Check sheet for the modelled part. Datum: model origin and axes. Units: mm. A direction names the side the tool comes from. Round coordinates to 2 decimals unless told otherwise and drop trailing zeros. Write each loop counter-clockwise with the first axis right and the second up, starting at its lowest first coordinate (ties: lowest second). Pieces come first, ordered by that corner, then holes. Notation, with made-up numbers: M 15.5,-14.75 L 67.5,-14.75 A24 ccw 67.5,-3.75 Z; hole C 83.25,76.5 d11. An arc over 180 degrees is marked long. Answer in a Markdown table with one row per item.
```python
from build123d import *

# Parameters (mm, degrees)
SKETCH1_W                    = 127
SKETCH1_H                    = 80.01
BASE_DEPTH                   = 3.81
SKETCH2_W                    = 127
SKETCH2_H                    = 3.81
FRONT_PANELING_DEPTH         = 76.2
SKETCH4_R                    = 1.651
ARDUINO_MOUNTING_HOLES_DEPTH = 107.95368168
STABILITY_STRUT_DEPTH        = 3.81
SKETCH5_R                    = 6.0325
ON_OFF_SWITCH_RECESS_DEPTH   = 130.751494018
SKETCH7_R                    = 3.683
SKETCH7_W                    = 1.778
SKETCH7_H                    = 3.81
POTENTIOMETER_RECESS_DEPTH   = 3.81


with BuildPart() as part:
    # Sketch1 → Base (new body)
    with BuildSketch(Plane(origin=(0, 0, 0), x_dir=(1, 0, 0), z_dir=(0, 1, 0))):
        Rectangle(SKETCH1_W, SKETCH1_H)
    extrude(amount=BASE_DEPTH)

    # Sketch2 → Front Paneling (add)
    with BuildSketch(Plane(origin=(0, 3.81, 0), x_dir=(1, 0, 0), z_dir=(0, 1, 0))):
        with Locations((0, -38.1)):
            Rectangle(SKETCH2_W, SKETCH2_H)
    extrude(amount=FRONT_PANELING_DEPTH)

    # Sketch4 → Arduino Mounting Holes (cut, through all)
    with BuildSketch(Plane(origin=(0, 3.81, 0), x_dir=(1, 0, 0), z_dir=(0, 1, 0))):
        with Locations(Location((-44.45, -28.575, 0), (0, 0, 270))):
            Circle(SKETCH4_R)
        with Locations(Location((-43.18, 19.685, 0), (0, 0, 270))):
            Circle(SKETCH4_R)
        with Locations(Location((31.75, 19.685, 0), (0, 0, 270))):
            Circle(SKETCH4_R)
        with Locations(Location((38.1, -28.575, 0), (0, 0, 270))):
            Circle(SKETCH4_R)
    extrude(amount=-ARDUINO_MOUNTING_HOLES_DEPTH, mode=Mode.SUBTRACT)

    # Sketch3 → Stability Strut (add)
    with BuildSketch(Plane.ZY.offset(55.88)):
        Polygon((36.195, 76.2), (-36.195, 3.81), (-31.115, 3.81), (36.195, 71.12), align=None)
    stability_strut = extrude(amount=STABILITY_STRUT_DEPTH)

    # Mirror Strut: Stability Strut across plane
    add(stability_strut.mirror(Plane(origin=(0, 0, 0), x_dir=(0, 0, 1), z_dir=(1, 0, 0))))

    # Sketch5 → On Off Switch Recess (cut, through all)
    with BuildSketch(Plane.XY.offset(40.005)):
        with Locations((44.45, 40.005)):
            Circle(SKETCH5_R)
    extrude(amount=-ON_OFF_SWITCH_RECESS_DEPTH, mode=Mode.SUBTRACT)

    # Sketch7 → Potentiometer Recess (cut)
    with BuildSketch(Plane.XY.offset(40.005)):
        with Locations((12.7, 40.005)):
            Circle(SKETCH7_R)
        with Locations((20.955, 40.005)):
            Rectangle(SKETCH7_W, SKETCH7_H)
    extrude(amount=-POTENTIOMETER_RECESS_DEPTH, mode=Mode.SUBTRACT)


solid = part.part
```
1. Draft check along Z on faces 1 (the face through (55.88, 37, 0)), 2 (the face through (-1, 39, 40.005)), 3 (the face through (36.488, 1.932, 28.217)), 4 (the face through (57.758, 40.512, 0.507)). Enter one of: +Z half, -Z half, draft (parallel to the pull), parting line (faces both ways), or undercut.
Found:
| item | result |
|---|---|
| face 1 | draft |
| face 2 | +Z half |
| face 3 | undercut |
| face 4 | -Z half |
2. Access from +Z, -Z, +X, -X, +Y, -Y to the whole of each face (thin tool, end or side, straight path). Record for faces 5 (the face through (57.758, 36.994, 2.069)), 6 (the face through (59.69, 37, 0)), 7 (the face through (20.066, 40, 38)), 8 (the face through (-55.88, 37, 0)).
Found:
| item | result |
|---|---|
| face 5 | +X, -X |
| face 6 | -Z, +X, +Y |
| face 7 | +Z, -Z |
| face 8 | -Z, +Y |
3. Section check D-D, the plane x = 44.45. Record the cut outline in (y, z) (1 decimal).
Found:
| item | result |
|---|---|
| outline | M 0,-40 L 3.8,-40 L 3.8,36.2 L 34,36.2 L 34,40 L 0,40 Z; M 46,36.2 L 80,36.2 L 80,40 L 46,40 Z |
4. Section check C-C, the plane z = 7. Record the cut outline in (x, y) (3 decimals), and give its area (3 significant figures).
Found:
| item | result |
|---|---|
| outline | M -63.5,0 L 63.5,0 L 63.5,3.81 L -63.5,3.81 Z; M -59.69,41.925 L -55.88,41.925 L -55.88,47.005 L -59.69,47.005 Z; M 55.88,41.925 L 59.69,41.925 L 59.69,47.005 L 55.88,47.005 Z |
| area | 523 mm2 |
5. Section check A-A, the plane x = 31.75. Record the cut outline in (y, z) (3 decimals).
Found:
| item | result |
|---|---|
| outline | M 0,-40.005 L 3.81,-40.005 L 3.81,-21.336 L 0,-21.336 Z; M 0,-18.034 L 3.81,-18.034 L 3.81,36.195 L 80.01,36.195 L 80.01,40.005 L 0,40.005 Z |
6. Go/stop test with flat-tipped pins: pin 1 (12 mm diameter, centred on y = 42.5, z = -5, fed in from +X); pin 2 (15.5 mm diameter, centred on x = 44.45, y = 40.005, fed in from -Z) (3 decimals); pin 3 (3 mm diameter, centred on x = 14, z = -8, fed in from +Y); pin 4 (2 mm diameter, centred on y = 24, z = -9, fed in from +X). Record where each tip stops, or that it passes through.
Found:
| item | result |
|---|---|
| pin 1 | stops at x = 59.69 |
| pin 2 | stops at z = 36.195 |
| pin 3 | stops at y = 3.81 |
| pin 4 | passes through |
7. Scan lines: L1, parallel to X at y = 18, z = -18.5; L2, parallel to Y at x = 44.45, z = 38; L3, parallel to Y at x = 0, z = -5. Record each from-to range of solid material in increasing order.
Found:
| item | result |
|---|---|
| L1 | x = -59.69 to -55.88, 55.88 to 59.69 |
| L2 | y = 0 to 33.97, 46.04 to 80.01 |
| L3 | y = 0 to 3.81 |
8. Section check B-B, the plane y = 28. Record the cut outline in (x, z) (3 decimals).
Found:
| item | result |
|---|---|
| outline | M -63.5,36.195 L 63.5,36.195 L 63.5,40.005 L -63.5,40.005 Z; M -59.69,-12.005 L -55.88,-12.005 L -55.88,-6.925 L -59.69,-6.925 Z; M 55.88,-12.005 L 59.69,-12.005 L 59.69,-6.925 L 55.88,-6.925 Z |
